from build123d import *

# Parameters (mm, degrees)
SKETCH_W   = 219
SKETCH_H   = 274
SKETCH_R   = 1.8
SKETCH_R_2 = 4.2
SKETCH_R_3 = 7.7
SKETCH_W_2 = 59.5
SKETCH_H_2 = 59.5
PAD_DEPTH  = 3


with BuildPart() as part:
    # Sketch → Pad (new body)
    with BuildSketch(Plane.XY):
        with Locations((0, 137)):
            Rectangle(SKETCH_W, SKETCH_H)
        with Locations((-104.5, 60)):
            Circle(SKETCH_R, mode=Mode.SUBTRACT)
        with Locations((104.5, 60)):
            Circle(SKETCH_R, mode=Mode.SUBTRACT)
        with Locations((-104.5, 269)):
            Circle(SKETCH_R, mode=Mode.SUBTRACT)
        with Locations((104.5, 269)):
            Circle(SKETCH_R, mode=Mode.SUBTRACT)
        with Locations((0, 35)):
            Circle(SKETCH_R_2, mode=Mode.SUBTRACT)
        with Locations((5.75, 29.25)):
            Circle(SKETCH_R, mode=Mode.SUBTRACT)
        with Locations((5.75, 40.75)):
            Circle(SKETCH_R, mode=Mode.SUBTRACT)
        with Locations((-5.75, 29.25)):
            Circle(SKETCH_R, mode=Mode.SUBTRACT)
        with Locations((-5.75, 40.75)):
            Circle(SKETCH_R, mode=Mode.SUBTRACT)
        with Locations((-58.485281, 23.485281)):
            Circle(SKETCH_R, mode=Mode.SUBTRACT)
        with Locations((-41.514719, 23.485281)):
            Circle(SKETCH_R, mode=Mode.SUBTRACT)
        with Locations((-41.514719, 6.514719)):
            Circle(SKETCH_R, mode=Mode.SUBTRACT)
        with Locations((-58.485281, 6.514719)):
            Circle(SKETCH_R, mode=Mode.SUBTRACT)
        with Locations((-50, 15)):
            Circle(SKETCH_R_3, mode=Mode.SUBTRACT)
        with Locations((41.514719, 23.485281)):
            Circle(SKETCH_R, mode=Mode.SUBTRACT)
        with Locations((58.485281, 23.485281)):
            Circle(SKETCH_R, mode=Mode.SUBTRACT)
        with Locations((58.485281, 6.514719)):
            Circle(SKETCH_R, mode=Mode.SUBTRACT)
        with Locations((41.514719, 6.514719)):
            Circle(SKETCH_R, mode=Mode.SUBTRACT)
        with Locations((50, 15)):
            Circle(SKETCH_R_3, mode=Mode.SUBTRACT)
        with Locations((-44.75, 209.25)):
            Rectangle(SKETCH_W_2, SKETCH_H_2, mode=Mode.SUBTRACT)
        with Locations((44.75, 209.25)):
            Rectangle(SKETCH_W_2, SKETCH_H_2, mode=Mode.SUBTRACT)
        with Locations((44.75, 119.75)):
            Rectangle(SKETCH_W_2, SKETCH_H_2, mode=Mode.SUBTRACT)
        with Locations((-44.75, 119.75)):
            Rectangle(SKETCH_W_2, SKETCH_H_2, mode=Mode.SUBTRACT)
    extrude(amount=PAD_DEPTH)


solid = part.part
Geometry: final body of the model. Coordinates: model frame, mm. Round coordinates to 2 decimals unless told otherwise and drop trailing zeros. Loops run counter-clockwise (first coordinate to the right, second up) from the corner with the lowest first, then second, coordinate; pieces in that order, holes last. Notation, with made-up numbers: M 45.5,54 L 90.5,54 A29 ccw 90.5,77 Z; hole C 29.25,14.25 d1. An arc over 180 degrees is marked long. Put each result on its own line as item: value. Start each with the question number.
(1) Contact query for a flat-ended pin moving along its axis: pin 1 Ø3 at (x, y) = (-41.51, 6.51) entering from -Z. Output: stop coordinate, or through.
(2) Draft query along X for faces 1 (the face through (-2, 139, 0)), 2 (the face through (2.26, 38.54, 1.48)). Return one class per face: +X half, -X half, draft (parallel to the pull), parting line (faces both ways), or undercut.
(3) Material intervals for line 1 along X through (y, z) = (193, 1.25); line 2 along Y through (x, z) = (-104.5, 2.2); line 3 along Y through (x, z) = (-29.5, 0.2), sorted ascending. Write a range as [from, to].
(4) Section query D-D (y = 101). Return loops of the section in (x, z).
(5) Section query A-A (x = -50). Return loops of the section in (y, z), then the cut area to 3 significant figures.
(6) Section query B-B (y = 35). Return loops of the section in (x, z), then the cut area to 3 significant figures.
(7) Section query C-C (x = 27). Return loops of the section in (y, z).
Findings below:
1. pin 1: passes through
2. face 1: draft
2. face 2: undercut
3. line 1: x = [-109.5, -74.5], [-15, 15], [74.5, 109.5]
3. line 2: y = [0, 58.2], [61.8, 267.2], [270.8, 274]
3. line 3: y = [0, 90], [149.5, 179.5], [239, 274]
4. outline: M -109.5,0 L -74.5,0 L -74.5,3 L -109.5,3 Z; M -15,0 L 15,0 L 15,3 L -15,3 Z; M 74.5,0 L 109.5,0 L 109.5,3 L 74.5,3 Z
5. outline: M 0,0 L 7.3,0 L 7.3,3 L 0,3 Z; M 22.7,0 L 90,0 L 90,3 L 22.7,3 Z; M 149.5,0 L 179.5,0 L 179.5,3 L 149.5,3 Z; M 239,0 L 274,0 L 274,3 L 239,3 Z
5. area: 419 mm2
6. outline: M -109.5,0 L -4.2,0 L -4.2,3 L -109.5,3 Z; M 4.2,0 L 109.5,0 L 109.5,3 L 4.2,3 Z
6. area: 632 mm2
7. outline: M 0,0 L 90,0 L 90,3 L 0,3 Z; M 149.5,0 L 179.5,0 L 179.5,3 L 149.5,3 Z; M 239,0 L 274,0 L 274,3 L 239,3 Z
